from build123d import *

# Parameters (mm, degrees)
SKETCH1_R                             = 79.375
BOSS_EXTRUDE1_DEPTH                   = 3.175
TAP_DRILL_FOR_M5X0_8_TAP1_D           = 4.2
TAP_DRILL_FOR_M7X1_0_TAP1_D           = 6
SKETCH32_R                            = 4
CUT_EXTRUDE1_DEPTH                    = 113.432663181
SKETCH32_4_R                          = 11
SKETCH32_4_R_2                        = 4
CUT_EXTRUDE2_DEPTH                    = 4.35
CHAMFER1_SIZE                         = 4.35
TAP_DRILL_FOR_M2X0_4_TAP1_D           = 1.6
TAP_DRILL_FOR_M2X0_4_TAP1_CSINK_D     = 1.65
TAP_DRILL_FOR_M2X0_4_TAP1_CSINK_ANGLE = 90
CHAMFER2_SIZE                         = 2.5
TAP_DRILL_FOR_M5X0_8_TAP2_D           = 4.2


with BuildPart() as part:
    # Sketch1 → Boss-Extrude1 (new, symmetric)
    with BuildSketch(Plane(origin=(0, 0, 0), x_dir=(1, 0, 0), z_dir=(0, 1, 0))):
        with Locations(Location((0, 0, 0), (0, 0, 270))):
            Circle(SKETCH1_R)
    extrude(amount=BOSS_EXTRUDE1_DEPTH, both=True)

    # Tap Drill for M5x0.8 Tap1 (through all)
    with Locations(Plane(origin=(0, 3.175, 0), x_dir=(1, 0, 0), z_dir=(0, 1, 0))):
        with Locations((-27.3188086, 41.38978387), (4.4311914, 41.38978387), (-15.875, -12.895910708), (15.875, -12.895910708)):
            Hole(TAP_DRILL_FOR_M5X0_8_TAP1_D / 2)

    # Tap Drill for M7x1.0 Tap1 (through all)
    with Locations(Plane(origin=(0, 3.175, 0), x_dir=(1, 0, 0), z_dir=(0, 1, 0))):
        with Locations((-44.245, 9.941583672), (-44.245, -15.058416328), (44.245, 9.941583672), (44.245, -15.058416328)):
            Hole(TAP_DRILL_FOR_M7X1_0_TAP1_D / 2)

    # Sketch32 → Cut-Extrude1 (cut, through all)
    with BuildSketch(Plane(origin=(0, 3.175, 0), x_dir=(1, 0, 0), z_dir=(0, 1, 0))):
        with Locations(Location((0, 0, 0), (0, 0, 270))):
            Circle(SKETCH32_R)
    extrude(amount=-CUT_EXTRUDE1_DEPTH, mode=Mode.SUBTRACT)

    # Sketch32<4> → Cut-Extrude2 (cut)
    with BuildSketch(Plane(origin=(0, 3.175, 0), x_dir=(1, 0, 0), z_dir=(0, 1, 0))):
        with Locations(Location((0, 0, 0), (0, 0, 270))):
            Circle(SKETCH32_4_R)
        with Locations(Location((0, 0, 0), (0, 0, 270))):
            Circle(SKETCH32_4_R_2, mode=Mode.SUBTRACT)
    extrude(amount=-CUT_EXTRUDE2_DEPTH, mode=Mode.SUBTRACT)

    # Chamfer1
    chamfer1_edges = [part.edges().sort_by_distance(p)[0] for p in [
        (0, 3.175, -11),
    ]]
    chamfer(chamfer1_edges, length=CHAMFER1_SIZE - 0.0001)  # a hair under: the kernel refuses the full size

    # Tap Drill for M2x0.4 Tap1 (through all)
    with Locations(Plane(origin=(0, -1.175, 0), x_dir=(1, 0, 0), z_dir=(0, 1, 0))):
        with Locations((-8, 0), (-5.656854249, 5.656854249), (0, 8), (5.656854249, 5.656854249), (8, 0), (5.656854249, -5.656854249), (0, -8), (-5.656854249, -5.656854249)):
            CounterSinkHole(TAP_DRILL_FOR_M2X0_4_TAP1_D / 2, TAP_DRILL_FOR_M2X0_4_TAP1_CSINK_D / 2, counter_sink_angle=TAP_DRILL_FOR_M2X0_4_TAP1_CSINK_ANGLE)

    # Chamfer2
    chamfer2_edges = [part.edges().sort_by_distance(p)[0] for p in [
        (0, 3.175, -79.375),
    ]]
    chamfer(chamfer2_edges, length=CHAMFER2_SIZE)

    # Tap Drill for M5x0.8 Tap2 (through all)
    with Locations(Plane(origin=(0, 3.175, 0), x_dir=(1, 0, 0), z_dir=(0, 1, 0))):
        with Locations((-57.723385101, 0), (0, 57.723385101), (57.723385101, 0), (0, -57.723385101)):
            Hole(TAP_DRILL_FOR_M5X0_8_TAP2_D / 2)


solid = part.part
Verification items for the finished model (mm, model axes). A direction names the side the tool comes from. Coordinates: 2 decimals unless noted, no trailing zeros. Use CSV: the item, a comma, the result in double quotes.
Q1. Go/stop test with flat-tipped pins: P1, Ø11, axis at x = -0.5, z = 3, coming from the +Y side (3 decimals); P2, Ø3, axis at y = -0.5, z = 39, coming from the +X side; P3, Ø1.5, axis at y = 0, z = 26.5, coming from the -X side. Record where each tip stops, or that it passes through.
Computed values:
P1,"y = -1.175"
P2,"x = 69.96"
P3,"x = -75.08"
Q2. Mould release check, pull along Z, two halves, no side actions. Record for faces 3 (the flat face through (1, -3.175, 17)), 4 (the cylindrical face through (23.84, -1.22, 75.71)), 5 (the cylindrical face through (0.455, -0.044, -55.673)): pulls with the +Z half, pulls with the -Z half, needs draft (parallel to the pull), parting line crosses it, or undercut.
Computed values:
face 3,"needs draft"
face 4,"parting line crosses it"
face 5,"undercut"
Q3. Set-up check for faces 1 (the cylindrical face through (46.63, -0.04, -8.12)), 2 (the flat face through (-5, -1.175, 0)): record each of +Z, -Z, +X, -X, +Y, -Y from which the full face is reachable in a straight line by a thin tool's end or side.
Computed values:
face 1,"+Y, -Y"
face 2,"+Y"
Q4. Thickness scan on line 1 along Z through (x, y) = (-47, -1.25); line 2 along Z through (x, y) = (45.5, -2.25); line 3 along X through (y, z) = (-2, -8). Record the ranges inside material, lowest first. Write a range as [from, to].
Computed values:
line 1,"[-63.96, -11.13], [-8.75, 13.87], [16.25, 63.96]"
line 2,"[-65.04, -12.67], [-7.22, 12.33], [17.78, 65.04]"
line 3,"[-78.97, -46.53], [-41.96, -0.8], [0.8, 41.96], [46.53, 78.97]"
